from build123d import *

# Parameters (mm, degrees)
SKETCH1_R               = 5
BOSS_EXTRUDE1_DEPTH     = 7.5
BOSS_EXTRUDE2_DEPTH     = 5
SKETCH3_R               = 2.46
CUT_EXTRUDE1_DEPTH      = 1
CUT_EXTRUDE1_DEPTH_BACK = 26
CHAMFER1_SIZE           = 0.5


with BuildPart() as part:
    # Sketch1 → Boss-Extrude1 (new body, symmetric)
    with BuildSketch(Plane.XY):
        Circle(SKETCH1_R)
    extrude(amount=BOSS_EXTRUDE1_DEPTH, both=True)

    # Sketch2 → Boss-Extrude2 (add)
    with BuildSketch(Plane.XY.offset(7.5)):
        Polygon((0.50159839, -4.59148477), (4.227141646, -1.861345437), (3.725543257, 2.730139333), (-0.50159839, 4.59148477), (-4.227141646, 1.861345437), (-3.725543257, -2.730139333), align=None)
    boss_extrude2 = extrude(amount=BOSS_EXTRUDE2_DEPTH)

    # Mirror1: Boss-Extrude2 across plane
    add(boss_extrude2.mirror(Plane.XY))

    # Sketch3 → Cut-Extrude1 (cut, two sides)
    with BuildSketch(Plane.XY.offset(12.5)) as cut_extrude1_sk:
        Circle(SKETCH3_R)
    extrude(amount=CUT_EXTRUDE1_DEPTH, mode=Mode.SUBTRACT)
    extrude(cut_extrude1_sk.sketch, amount=-CUT_EXTRUDE1_DEPTH_BACK, mode=Mode.SUBTRACT)

    # Chamfer1
    chamfer1_edges = [part.edges().sort_by_distance(p)[0] for p in [
        (-2.46, 0, 12.5),
        (-2.46, 0, -12.5),
    ]]
    chamfer(chamfer1_edges, length=CHAMFER1_SIZE)

    # Sketch8 → Cut-Revolve3 (revolve, cut)
    with BuildSketch(Plane(origin=(0, 0, 0), x_dir=(-0.915203013, 0.402993108, 0), z_dir=(-0.402993108, -0.915203013, 0))):
        Polygon((4, 12.5), (4.618802154, 12.5), (4.618802154, 11.881197846), align=None)
    cut_revolve3 = revolve(axis=Axis((0, 0, -12), (0, 0, 1)), mode=Mode.SUBTRACT)

    # Mirror2: Cut-Revolve3 across plane
    add(cut_revolve3.mirror(Plane.XY), mode=Mode.SUBTRACT)


solid = part.part
Source: CAD feature listing. Evaluate the final solid. Frame: model axes, mm. A direction names the side the tool comes from. Give positions to 0.01 mm unless a question says otherwise; leave off trailing zeros. Loops run counter-clockwise (first coordinate to the right, second up) from the corner with the lowest first, then second, coordinate; pieces in that order, holes last. Notation, with made-up numbers: (-31, 77) -> (28, 77) arc R21 cw to (28, 91) -> close; hole circle Ø8 at (-10, 44.25). An arc over 180 degrees is marked (long way). Use a Markdown table: item, result. Add a question column.
1) Line query: line 1 along Y through (x, z) = (0, -2.5); line 2 along Z through (x, y) = (-0.5, -4.25); line 3 along X through (y, z) = (-0.25, 8.25). Output: solid intervals per line, ascending. Write a range as [from, to].
2) Reachability of faces 1 (the face through (3.98, 0.4, 9.96)), 2 (the face through (1.64, 3.65, -9.96)), 3 (the face through (2, -4, 7.5)), 4 (the face through (2.338, -3.246, 9.965)), 5 (the face through (-1.64, -3.65, -9.96)) from +Z, -Z, +X, -X, +Y, -Y: full face, straight path, thin tool, end or side. Return the list, or none.
3) Section query C-C, the plane x = 0. Return the cut outline in (y, z), then the cut area to 3 significant figures.
4) Pull-direction query (Y, two-part tool) for faces 6 (the face through (2.272, -0.942, 0.168)), 7 (the face through (-0.44, 4.124, 12.352)), 8 (the face through (1, 3, -12.5)); classes: +Y half, -Y half, draft (parallel to the pull), parting line (faces both ways), or undercut.
5) Section query D-D, the plane z = 5.5. Return the cut outline in (x, y).
6) Section query A-A, the plane z = 8.5. Return the cut outline in (x, y).
7) First-contact query: pin 1 (5.5 mm diameter, centred on x = 0, y = 0, fed in from -Z); pin 2 (1.5 mm diameter, centred on x = 2.5, z = -9.5, fed in from +Y); pin 3 (1 mm diameter, centred on x = -3, z = -1.5, fed in from +Y). Flat tips, straight axial feed; report the tip coordinate or a pass-through.
Numbers:
| question | item | result |
|---|---|---|
| 1 | line 1 | y = [-5, -2.46], [2.46, 5] |
| 1 | line 2 | z = [-7.5, 7.5] |
| 1 | line 3 | x = [-4, -2.45], [2.45, 4.05] |
| 2 | face 1 | +Z, +X, +Y |
| 2 | face 2 | -Z, +X, +Y |
| 2 | face 3 | +Z |
| 2 | face 4 | +Z, +X, -Y |
| 2 | face 5 | -Z, -X, -Y |
| 3 | outline | (-5, -7.5) -> (-4.37, -7.5) -> (-4.37, -12.13) -> (-4, -12.5) -> (-2.96, -12.5) -> (-2.46, -12) -> (-2.46, 12) -> (-2.96, 12.5) -> (-4, 12.5) -> (-4.37, 12.13) -> (-4.37, 7.5) -> (-5, 7.5) -> close; (2.46, -12) -> (2.96, -12.5) -> (4, -12.5) -> (4.37, -12.13) -> (4.37, -7.5) -> (5, -7.5) -> (5, 7.5) -> (4.37, 7.5) -> (4.37, 12.13) -> (4, 12.5) -> (2.96, 12.5) -> (2.46, 12) -> close |
| 3 | area | 114 mm2 |
| 4 | face 6 | undercut |
| 4 | face 7 | +Y half |
| 4 | face 8 | draft |
| 5 | outline | circle Ø10 at (0, 0); hole circle Ø4.92 at (0, 0) |
| 6 | outline | (-4.23, 1.86) -> (-3.73, -2.73) -> (0.5, -4.59) -> (4.23, -1.86) -> (3.73, 2.73) -> (-0.5, 4.59) -> close; hole circle Ø4.92 at (0, 0) |
| 7 | pin 1 | stops at z = -12.29 |
| 7 | pin 2 | stops at y = 3.6 |
| 7 | pin 3 | stops at y = 4.33 |
